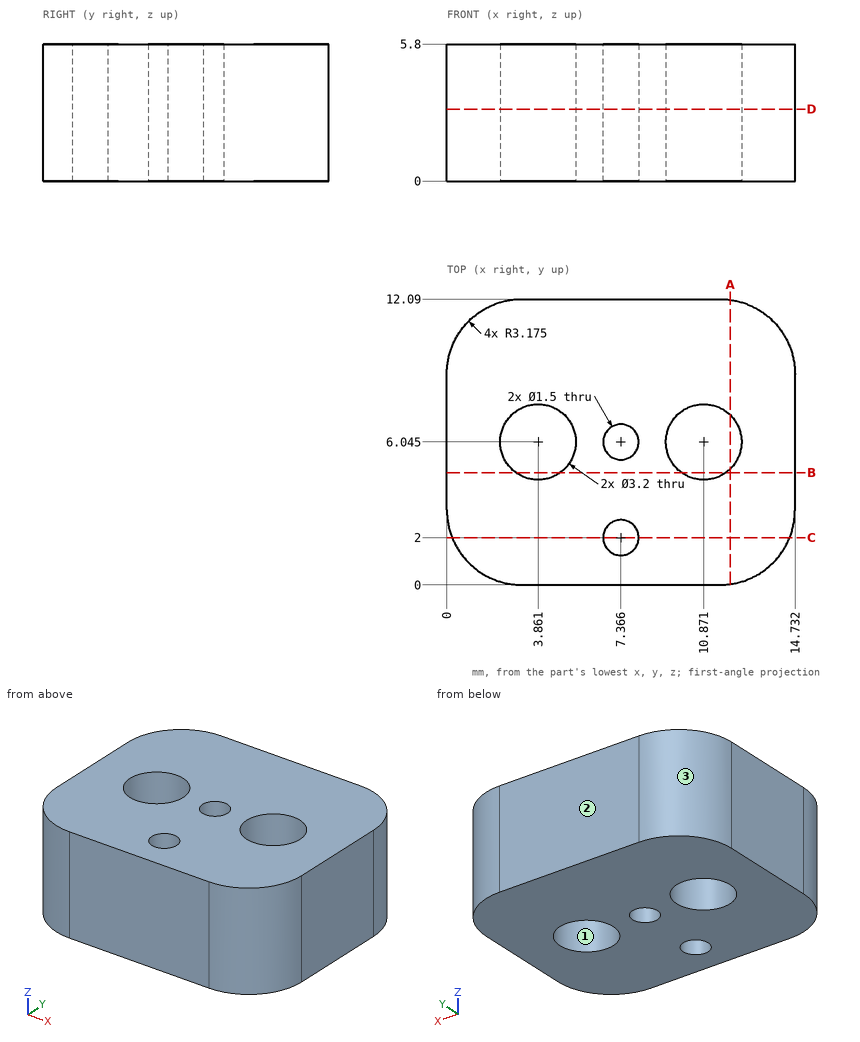
Check sheet for the drawn part. Datum: minimum x, y, z corner. Units: mm. Coordinates: 2 decimals unless noted, no trailing zeros. Order: outer loops, then holes, each group sorted by start corner. A loop starts at its lowest first (then second) coordinate and runs counter-clockwise, first axis right, second up. Notation, with made-up numbers: M -13.75,-37 L 12.25,-37 A24 cw 12.25,-7 Z; hole C 55,29 d8. An arc over 180 degrees is marked long. One line per item, written item: value. Start each with the question number.
Item 1: Sectioned sample at D-D (z = 3.05). Count the separate pieces of the cut face and the enclosed holes in it, then the cut area to 3 significant figures.
Item 2: Sectioned sample at B-B (y = 4.75). Enter the section's corners in (x, z).
Item 3: Scan lines: probe 1 along X at (y, z) = (6, 5) (1 decimal); probe 2 along X at (y, z) = (6.25, 3.3) (1 decimal); probe 3 along Y at (x, z) = (12.25, 1.45) (1 decimal). Record each from-to range of solid material in increasing order.
Item 4: Mould release check, pull along X, two halves, no side actions. Record for the marked faces 1, 2 and 3: released by +X, released by -X, zero draft, split by the parting line, or undercut.
Item 5: Sectioned sample at C-C (y = 2). Enter the section's corners in (x, z) (1 decimal).
Item 6: Sectioned sample at A-A (x = 12). Enter the section's corners in (y, z).
Item 7: Gauge pin test, flat end, axial feed: pin 1 (0.9 mm diameter, centred on x = 7.366, y = 2, fed in from -Z). Record the tip position at first contact, or that the pin passes through.
Conclusion:
1. separate pieces: 1
1. enclosed holes: 4
1. area: 150 mm^2
2. outline: M 0,0 L 2.92,0 L 2.92,5.8 L 0,5.8 Z; M 4.8,0 L 9.93,0 L 9.93,5.8 L 4.8,5.8 Z; M 11.81,0 L 14.73,0 L 14.73,5.8 L 11.81,5.8 Z
3. probe 1: x = 0 to 2.3, 5.5 to 6.6, 8.1 to 9.3, 12.5 to 14.7
3. probe 2: x = 0 to 2.3, 5.4 to 6.6, 8.1 to 9.3, 12.5 to 14.7
3. probe 3: y = 0.1 to 5.2, 6.9 to 12
4. face 1: undercut
4. face 2: zero draft
4. face 3: released by -X
5. outline: M 0.2,0 L 6.6,0 L 6.6,5.8 L 0.2,5.8 Z; M 8.1,0 L 14.5,0 L 14.5,5.8 L 8.1,5.8 Z
6. outline: M 0.03,0 L 4.91,0 L 4.91,5.8 L 0.03,5.8 Z; M 7.18,0 L 12.06,0 L 12.06,5.8 L 7.18,5.8 Z
7. pin 1: passes through
